For this review, take the finished solid that the model builds, in its own axes (mm). Coordinates: 2 decimals unless noted, no trailing zeros. Loops run counter-clockwise (first coordinate to the right, second up) from the corner with the lowest first, then second, coordinate; pieces in that order, holes last. Notation, with made-up numbers: M 1.25,32 L 59.25,32 A36 ccw 59.25,67 Z; hole C 59.25,46 d10. An arc over 180 degrees is marked long. Write each question's results on one line, items separated by ' | '. Start each with the question number.
```python
from build123d import *
from build123d.topology import SkipClean

# Parameters (mm, degrees)
BOSS_EXTRUDE1_DEPTH      = 160
CUT_EXTRUDE1_REACH       = 173.674
CUT_EXTRUDE1_END_RADIUS  = 44
SKETCH2_R                = 1.85
BOSS_EXTRUDE2_DEPTH      = 7.5
BOSS_EXTRUDE2_DEPTH_BACK = 7.5
CUT_EXTRUDE2_START       = -160
SKETCH5_W                = 1.237164205
SKETCH5_H                = 7.554303916
CUT_EXTRUDE2_DEPTH       = 160
SKETCH6_W                = 160
SKETCH6_H                = 7.554303916
SKETCH6_R                = 1.85
BOSS_EXTRUDE3_DEPTH      = 0.5
BOSS_EXTRUDE4_DEPTH      = 85
FILLET3_R                = 0.5
CUT_EXTRUDE4_REACH       = 176.326
CUT_EXTRUDE4_END_RADIUS  = 44
SKETCH9_W                = 12
SKETCH9_H                = 6
CUT_EXTRUDE5_DEPTH       = 72
CUT_EXTRUDE6_START       = -160
CUT_EXTRUDE6_DEPTH       = 160
BOSS_EXTRUDE5_DEPTH      = 1
BOSS_EXTRUDE5_DEPTH_BACK = 1.5
SKETCH14_W               = 160
SKETCH14_H               = 7.554303916
SKETCH14_R               = 1.85
SKETCH17_W               = 0.3144145
SKETCH17_H               = 160
CUT_EXTRUDE8_DEPTH       = 7.554303916
FILLET4_R                = 10
SKETCH18_W               = 5.679513367
SKETCH18_H               = 15.054755776
CUT_EXTRUDE9_DEPTH       = 15
CUT_EXTRUDE10_REACH      = 211.375
CUT_EXTRUDE10_END_RADIUS = 44
CUT_EXTRUDE10_START      = 20
SKETCH19_R               = 1.5
BOSS_EXTRUDE6_DEPTH      = 13


with BuildPart() as part:
    # Sketch1 → Boss-Extrude1 (new body)
    with BuildSketch(Plane.XY):
        with BuildLine():
            Line((-44, 0), (-42.75, 0))
            ThreePointArc((-42.75, 0), (0, -42.75), (42.75, 0))
            Line((42.75, 0), (44, 0))
            ThreePointArc((44, 0), (0, -44), (-44, 0))
        make_face()
    extrude(amount=BOSS_EXTRUDE1_DEPTH)

    # Cut-Extrude1: up to this cylinder (the profile starts inside it)
    cut_extrude1_end = Plane(origin=(0, 0, 80), z_dir=(0, 0, -1)) * Cylinder(CUT_EXTRUDE1_END_RADIUS, 571.348, mode=Mode.PRIVATE)
    # Sketch2 → Cut-Extrude1 (cut, up to the surface)
    with BuildSketch(Plane(origin=(0, 0, 0), x_dir=(0, 0, -1), z_dir=(1, 0, 0)), mode=Mode.PRIVATE) as cut_extrude1_sk1:
        with Locations((-147.5, -5)):
            Circle(SKETCH2_R)
    cut_extrude1_tool1 = extrude(cut_extrude1_sk1.sketch, amount=-CUT_EXTRUDE1_REACH, mode=Mode.PRIVATE) & cut_extrude1_end
    add(cut_extrude1_tool1.solids().sort_by_distance((0, -5, 147.5))[0], mode=Mode.SUBTRACT)
    # Sketch2 → Cut-Extrude1 (cut, up to the surface)
    with BuildSketch(Plane(origin=(0, 0, 0), x_dir=(0, 0, -1), z_dir=(1, 0, 0)), mode=Mode.PRIVATE) as cut_extrude1_sk2:
        with Locations((-115.5, -5)):
            Circle(SKETCH2_R)
    cut_extrude1_tool2 = extrude(cut_extrude1_sk2.sketch, amount=-CUT_EXTRUDE1_REACH, mode=Mode.PRIVATE) & cut_extrude1_end
    add(cut_extrude1_tool2.solids().sort_by_distance((0, -5, 115.5))[0], mode=Mode.SUBTRACT)
    # Sketch2 → Cut-Extrude1 (cut, up to the surface)
    with BuildSketch(Plane(origin=(0, 0, 0), x_dir=(0, 0, -1), z_dir=(1, 0, 0)), mode=Mode.PRIVATE) as cut_extrude1_sk3:
        with Locations((-44.5, -5)):
            Circle(SKETCH2_R)
    cut_extrude1_tool3 = extrude(cut_extrude1_sk3.sketch, amount=-CUT_EXTRUDE1_REACH, mode=Mode.PRIVATE) & cut_extrude1_end
    add(cut_extrude1_tool3.solids().sort_by_distance((0, -5, 44.5))[0], mode=Mode.SUBTRACT)
    # Sketch2 → Cut-Extrude1 (cut, up to the surface)
    with BuildSketch(Plane(origin=(0, 0, 0), x_dir=(0, 0, -1), z_dir=(1, 0, 0)), mode=Mode.PRIVATE) as cut_extrude1_sk4:
        with Locations((-12.5, -5)):
            Circle(SKETCH2_R)
    cut_extrude1_tool4 = extrude(cut_extrude1_sk4.sketch, amount=-CUT_EXTRUDE1_REACH, mode=Mode.PRIVATE) & cut_extrude1_end
    add(cut_extrude1_tool4.solids().sort_by_distance((0, -5, 12.5))[0], mode=Mode.SUBTRACT)

    # Sketch4 → Boss-Extrude2 (add, two sides: drawn at the far end of the back side and taken through both)
    with SkipClean():  # the faces are left unmerged after this step: merging them gives an invalid solid
        with BuildSketch(Plane(origin=(0, 0, 72), x_dir=(-1, 0, 0), z_dir=(0, 0, -1)).offset(-BOSS_EXTRUDE2_DEPTH_BACK)):
            with BuildLine():
                Line((-42.188440557, 12.495418496), (-40.883089617, 12.495418496))
                ThreePointArc((-40.883089617, 12.495418496), (-42.280696429, 6.317057024), (-42.75, 0))
                Line((-42.75, 0), (-44, 0))
                ThreePointArc((-44, 0), (-43.544755049, 6.31302683), (-42.188440557, 12.495418496))
            make_face()
        extrude(amount=BOSS_EXTRUDE2_DEPTH + BOSS_EXTRUDE2_DEPTH_BACK)

    # Sketch5 → Cut-Extrude2 (cut)
    with SkipClean():  # the faces are left unmerged after this step: merging them gives an invalid solid
        with BuildSketch(Plane.XY.offset(160).offset(CUT_EXTRUDE2_START)):
            with Locations((-43.381417898, -3.777151958)):
                Rectangle(SKETCH5_W, SKETCH5_H)
        extrude(amount=CUT_EXTRUDE2_DEPTH, mode=Mode.SUBTRACT)

    # Sketch6 → Boss-Extrude3 (add)
    with SkipClean():  # the faces are left unmerged after this step: merging them gives an invalid solid
        with BuildSketch(Plane.ZY.offset(42.762835795)):
            with Locations((80, -3.777151958)):
                Rectangle(SKETCH6_W, SKETCH6_H)
            with Locations((12.5, -5)):
                Circle(SKETCH6_R, mode=Mode.SUBTRACT)
            with Locations((44.5, -5)):
                Circle(SKETCH6_R, mode=Mode.SUBTRACT)
            with Locations((115.5, -5)):
                Circle(SKETCH6_R, mode=Mode.SUBTRACT)
            with Locations((147.5, -5)):
                Circle(SKETCH6_R, mode=Mode.SUBTRACT)
        extrude(amount=BOSS_EXTRUDE3_DEPTH)

    # Sketch7 → Boss-Extrude4 (add)
    with SkipClean():  # the faces are left unmerged after this step: merging them gives an invalid solid
        with BuildSketch(Plane.XY.offset(160)):
            with BuildLine():
                Line((3.193641617, -47.271567965), (4.247348412, -46.182404151))
                ThreePointArc((4.247348412, -46.182404151), (-1.361382554, -53.250007087), (-2.652595344, -44.320189404))
                Line((-2.652595344, -44.320189404), (-7.064595581, -42.922505627))
                ThreePointArc((-7.064595581, -42.922505627), (0, -43.5), (7.064595581, -42.922505627))
                Line((7.064595581, -42.922505627), (2.652595344, -44.320189404))
                Line((2.652595344, -44.320189404), (-0.081202248, -45.006637866))
                ThreePointArc((-0.081202248, -45.006637866), (-2.072088401, -51.385243836), (3.193641617, -47.271567965))
            make_face()
        extrude(amount=-BOSS_EXTRUDE4_DEPTH)

    # Fillet3
    fillet3_edges = [part.edges().sort_by_distance(p)[0] for p in [
        (4.247348412, -46.182404151, 117.5),
    ]]
    fillet(fillet3_edges, radius=FILLET3_R)

    # Cut-Extrude4: up to this cylinder (the profile starts inside it)
    with SkipClean():  # the faces are left unmerged after this step: merging them gives an invalid solid
        cut_extrude4_end = Plane(origin=(0, 0, 72), z_dir=(0, 0, -1)) * Cylinder(CUT_EXTRUDE4_END_RADIUS, 441.652, mode=Mode.PRIVATE)
        # Sketch9 → Cut-Extrude4 (cut, up to the surface)
        with BuildSketch(Plane(origin=(0, 0, 0), x_dir=(0, 0, -1), z_dir=(1, 0, 0)), mode=Mode.PRIVATE) as cut_extrude4_sk1:
            with Locations((-72, 5.495418496)):
                Rectangle(SKETCH9_W, SKETCH9_H)
        cut_extrude4_tool1 = extrude(cut_extrude4_sk1.sketch, amount=CUT_EXTRUDE4_REACH, mode=Mode.PRIVATE) & cut_extrude4_end
        add(cut_extrude4_tool1.solids().sort_by_distance((0, 5.495418, 72))[0], mode=Mode.SUBTRACT)

    # Sketch11 → Cut-Extrude5 (cut)
    with SkipClean():  # the faces are left unmerged after this step: merging them gives an invalid solid
        with BuildSketch(Plane.XY.offset(160)):
            with BuildLine():
                Line((6.038191003, -53.758519386), (4.340910446, -43.785345682))
                ThreePointArc((4.340910446, -43.785345682), (0, -44), (-4.340910446, -43.785345682))
                Line((-4.340910446, -43.785345682), (-6.663752415, -46.7537351))
                ThreePointArc((-6.663752415, -46.7537351), (-2.196447495, -53.671825429), (6.038191003, -53.758519386))
            make_face()
        extrude(amount=-CUT_EXTRUDE5_DEPTH, mode=Mode.SUBTRACT)

    # Sketch12 → Cut-Extrude6 (cut)
    with SkipClean():  # the faces are left unmerged after this step: merging them gives an invalid solid
        with BuildSketch(Plane(origin=(0, 0, 0), x_dir=(-1, 0, 0), z_dir=(0, 0, -1)).offset(CUT_EXTRUDE6_START)):
            Polygon((42.75, 0), (42.75, -7.554303916), (41.523020522, -7.554303916), align=None)
        extrude(amount=CUT_EXTRUDE6_DEPTH, mode=Mode.SUBTRACT)

    # Sketch14 → Boss-Extrude5 (add, two sides: drawn at the far end of the back side and taken through both)
    with SkipClean():  # the faces are left unmerged after this step: merging them gives an invalid solid
        with BuildSketch(Plane.ZY.offset(43.262835795).offset(-BOSS_EXTRUDE5_DEPTH_BACK)):
            with Locations((80, -3.777151958)):
                Rectangle(SKETCH14_W, SKETCH14_H)
            with Locations((12.5, -5)):
                Circle(SKETCH14_R, mode=Mode.SUBTRACT)
            with Locations((44.5, -5)):
                Circle(SKETCH14_R, mode=Mode.SUBTRACT)
            with Locations((115.5, -5)):
                Circle(SKETCH14_R, mode=Mode.SUBTRACT)
            with Locations((147.5, -5)):
                Circle(SKETCH14_R, mode=Mode.SUBTRACT)
        extrude(amount=BOSS_EXTRUDE5_DEPTH + BOSS_EXTRUDE5_DEPTH_BACK)

    # Sketch17 → Cut-Extrude8 (cut)
    with SkipClean():  # the faces are left unmerged after this step: merging them gives an invalid solid
        with BuildSketch(Plane.XZ.offset(7.554303916)):
            with Locations((-41.920043045, 80)):
                Rectangle(SKETCH17_W, SKETCH17_H)
        extrude(amount=-CUT_EXTRUDE8_DEPTH, mode=Mode.SUBTRACT)

    # Fillet4
    # the kernel refuses this fillet: 10 mm, written as the material it adds along each edge
    with BuildSketch(Plane(origin=(-43.346654915, -7.554303916, 160), x_dir=(0.21136107775555732, -0.9774080492864836, 0), z_dir=(0, 0, -1))) as fillet4_piece_1:
        with BuildLine():
            CenterArc((3.960443366, 9.991830737), FILLET4_R, 245.454934631, 22.228958211)
            Line((-0.193644978, 0.895482567), (-0.276726745, 0.713555603))
            ThreePointArc((-0.276726745, 0.713555603), (-0.292304099, 0.405469068), (-0.19548161, -0.042272216))
            Line((-0.19548161, -0.042272216), (0.008082537, -0.199836615))
            ThreePointArc((0.008082537, -0.199836615), (1.778158246, -0.164055241), (3.548233954, -0.199836615))
            Line((3.548233954, -0.199836615), (3.556316492, 0))
        make_face()
    extrude(amount=160)

    # Sketch18 → Cut-Extrude9 (cut)
    with BuildSketch(Plane.XY.offset(79.5)):
        with Locations((42.974138408, 7.527377888)):
            Rectangle(SKETCH18_W, SKETCH18_H)
    extrude(amount=-CUT_EXTRUDE9_DEPTH, mode=Mode.SUBTRACT)

    # Cut-Extrude10: up to this cylinder (the profile starts inside it)
    cut_extrude10_end = Plane(origin=(0, 0, 80), z_dir=(0, 0, -1)) * Cylinder(CUT_EXTRUDE10_END_RADIUS, 526.75, mode=Mode.PRIVATE)
    # Sketch19 → Cut-Extrude10 (cut, up to the surface)
    with BuildSketch(Plane(origin=(-42.077250295, 0, 0), x_dir=(0, 0, -1), z_dir=(1, 0, 0)).offset(CUT_EXTRUDE10_START), mode=Mode.PRIVATE) as cut_extrude10_sk1:
        with Locations(Location((-87.5, -15, 0), (0, 0, 180))):
            Circle(SKETCH19_R)
    cut_extrude10_tool1 = extrude(cut_extrude10_sk1.sketch, amount=CUT_EXTRUDE10_REACH, mode=Mode.PRIVATE) & cut_extrude10_end
    add(cut_extrude10_tool1.solids().sort_by_distance((-22.07725, -15, 87.5))[0], mode=Mode.SUBTRACT)
    # Sketch19 → Cut-Extrude10 (cut, up to the surface)
    with BuildSketch(Plane(origin=(-42.077250295, 0, 0), x_dir=(0, 0, -1), z_dir=(1, 0, 0)).offset(CUT_EXTRUDE10_START), mode=Mode.PRIVATE) as cut_extrude10_sk2:
        with Locations(Location((-72.5, -15, 0), (0, 0, 180))):
            Circle(SKETCH19_R)
    cut_extrude10_tool2 = extrude(cut_extrude10_sk2.sketch, amount=CUT_EXTRUDE10_REACH, mode=Mode.PRIVATE) & cut_extrude10_end
    add(cut_extrude10_tool2.solids().sort_by_distance((-22.07725, -15, 72.5))[0], mode=Mode.SUBTRACT)

    # Sketch20 → Boss-Extrude6 (add)
    with BuildSketch(Plane(origin=(0, 0, 75), x_dir=(-1, 0, 0), z_dir=(0, 0, -1))):
        with BuildLine():
            Line((4.237574899, -51.126366777), (9.364668734, -42.991894347))
            ThreePointArc((9.364668734, -42.991894347), (6.86426372, -43.461268776), (4.340910446, -43.785345682))
            Line((4.340910446, -43.785345682), (2.652595344, -44.320189404))
            ThreePointArc((2.652595344, -44.320189404), (4.866254034, -47.392325259), (4.237574899, -51.126366777))
        make_face()
    extrude(amount=-BOSS_EXTRUDE6_DEPTH)


solid = part.part
```
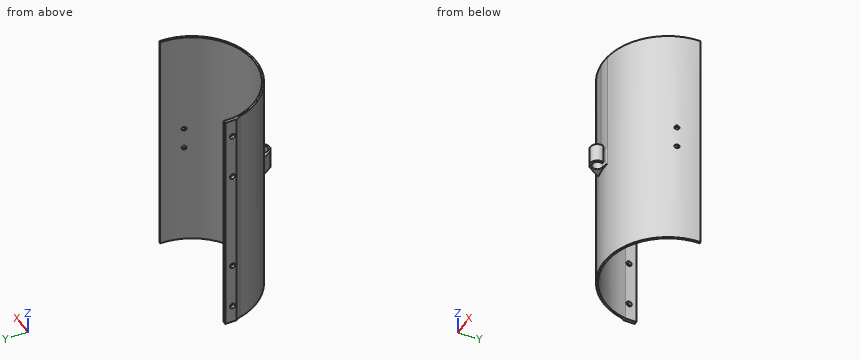
Q1. Take a section at C-C, the plane y = -32.5. Give the boundary of the cut face in (x, z).
Q2. Take a section at D-D, the plane z = 38. Give the boundary of the cut face in (x, y), then the cut area to 3 significant figures.
Q3. To check wall thickness, follow line 1 along Z through (x, y) = (-43.45, -5); line 2 along Z through (x, y) = (41, -15); line 3 along X through (y, z) = (-34, 133.5). State the ranges of each line that lie inside material, in increasing order.
Q4. Take a section at B-B, the plane y = -5. Give the boundary of the cut face in (x, z).
Q5. Take a section at A-A, the plane z = 115.5. Give the boundary of the cut face in (x, y).
Q6. Insertion check: P1, Ø2, axis at x = -33.5, z = 124, coming from the -Y side; P2, Ø1, axis at x = -4, y = -44.5, coming from the -Z side; P3, Ø3, axis at x = -11.5, z = 125, coming from the +Y side. Each pin has a flat end and moves straight along its axis. Give the tip position at first contact, or say it passes through.
Results:
1) outline: M -29.66,0 L -27.77,0 L -27.77,160 L -29.66,160 Z; M 27.77,0 L 29.66,0 L 29.66,160 L 27.77,160 Z
2) outline: M -44.26,-7.55 A10 cw -42.59,-11.03 A44 ccw 44,0 L 42.75,0 A42.75 cw -42.08,-7.55 L -42.08,0 L -44.26,0 Z | area: 178 mm^2
3) line 1: 0 to 10.65, 14.35 to 42.65, 46.35 to 113.65, 117.35 to 145.65, 149.35 to 160 | line 2: 0 to 71, 74 to 86, 89 to 160 | line 3: -27.93 to -25.91, 25.91 to 27.93
4) outline: M -44.26,0 L -42.08,0 L -42.08,10.65 L -44.26,10.65 Z; M -44.26,14.35 L -42.08,14.35 L -42.08,42.65 L -44.26,42.65 Z; M -44.26,46.35 L -42.08,46.35 L -42.08,113.65 L -44.26,113.65 Z; M -44.26,117.35 L -42.08,117.35 L -42.08,145.65 L -44.26,145.65 Z; M -44.26,149.35 L -42.08,149.35 L -42.08,160 L -44.26,160 Z; M 42.46,0 L 43.71,0 L 43.71,160 L 42.46,160 Z
5) outline: M -44.26,-7.55 A10 cw -42.59,-11.03 A44 ccw 44,0 L 42.75,0 A42.75 cw -42.08,-7.55 L -42.08,-6.85 L -44.26,-6.85 Z; M -44.26,-3.15 L -42.08,-3.15 L -42.08,0 L -44.26,0 Z
6) P1: y = -29.66 | P2: z = 75 | P3: y = -40.73
